Geometry check sheet. Reference: the model listing, model coordinates, mm. A direction names the side the tool comes from. Round coordinates to 2 decimals unless told otherwise and drop trailing zeros. Loops run counter-clockwise (first coordinate to the right, second up) from the corner with the lowest first, then second, coordinate; pieces in that order, holes last. Notation, with made-up numbers: (47, -8) - (83, -8) arc R23 cw to (83, 18) - close; hole circle Ø7 at (29.5, -4). An arc over 180 degrees is marked (long way). Answer in a Markdown table with one row per item. Add a question column.
```python
from build123d import *

# Parameters (mm, degrees)
F0_R     = 10
F1_DEPTH = 2
F2_R     = 4
F3_DEPTH = 0.5
F4_R     = 3.175
F5_DEPTH = 2
F6_R     = 9
F6_R_2   = 8
F6_R_3   = 7
F6_R_4   = 6
F6_R_5   = 5
F6_R_6   = 4
F7_DEPTH = 0.5
F8_SIZE2 = 0.49999
F8_SIZE  = 5.99999
F9_SIZE  = 0.5


# Not quite as in the source:
# - a fillet or chamfer is up to 0.001 mm smaller than in the source, because OpenCascade refuses the exact size


with BuildPart() as f1:
    # F0 (on Top) → F1 (new body)
    with BuildSketch(Plane.XY):
        Circle(F0_R)
    extrude(amount=F1_DEPTH)

    # F2 (on face) → F3 (join)
    with BuildSketch(Plane.XY.offset(2)):
        Circle(F2_R)
    extrude(amount=F3_DEPTH)

    # F4 (on face) → F5 (join)
    with BuildSketch(Plane.XY.offset(2.5)):
        Circle(F4_R)
    extrude(amount=F5_DEPTH)

    # F6 (on face) → F7 (cut)
    with BuildSketch(Plane(origin=(0, 0, 0), x_dir=(1, 0, 0), z_dir=(0, 0, -1))):
        Circle(F6_R)
        Circle(F6_R_2, mode=Mode.SUBTRACT)
        Circle(F6_R_3)
        Circle(F6_R_4, mode=Mode.SUBTRACT)
        Circle(F6_R_5)
        Circle(F6_R_6, mode=Mode.SUBTRACT)
    extrude(amount=-F7_DEPTH, mode=Mode.SUBTRACT)

    # F8 (size 6 and 0.5 in the source; OpenCascade refuses exactly that, so slightly less here)
    f8_edges = [f1.edges().sort_by_distance(p)[0] for p in [
        (-10, 0, 2),
    ]]
    f8_side = f1.faces().sort_by_distance((-9.717157, 0, 2))[0]
    chamfer(f8_edges, length=F8_SIZE, length2=F8_SIZE2, reference=f8_side)

    # F9
    f9_edges = [f1.edges().sort_by_distance(p)[0] for p in [
        (-3.175, 0, 4.5),
    ]]
    chamfer(f9_edges, length=F9_SIZE)


solid = f1.part
```
Q1. Cross-section at A-A, the plane z = 2.8. Enter the section's corners in (x, y) (3 decimals), plus the area to 3 significant figures.
Q2. Set-up check for faces 1 (the cylindrical face through (-0.69, -3.1, 3.24)), 2 (the flat face through (4, -6, 0)), 3 (the cylindrical face through (-1.08, 4.88, 0.25)): record each of +Z, -Z, +X, -X, +Y, -Y from which the full face is reachable in a straight line by a thin tool's end or side.
Q3. Depth check by flat-ended pin: P1, Ø9, axis at x = -2, y = -1, coming from the -Z side; P2, Ø2, axis at x = -1.5, z = 1, coming from the -Y side. Enter the tip coordinate at first touch or a pass-through.
Q4. Scan lines: line 1 (Z direction, x = 4, y = 0.75); line 2 (Z direction, x = -3.5, y = 0.25); line 3 (Y direction, x = 2.25, z = 2.7). Record each from-to range of solid material in increasing order. Write a range as from..to.
Q5. Release check for a two-part mould opening along X. For faces 4 (the conical face through (4.17, 1.31, 1.97)), 5 (the flat face through (-3, 2, 2.5)), 6 (the cylindrical face through (6.466, 2.681, 0.246)) record: +X half, -X half, draft (parallel to the pull), parting line (faces both ways), or undercut.
Check sheet entries:
| question | item | result |
|---|---|---|
| 1 | outline | circle Ø6.35 at (0, 0) |
| 1 | area | 31.7 mm² |
| 2 | face 1 | +Z |
| 2 | face 2 | -Z, +X, -X, +Y, -Y |
| 2 | face 3 | -Z |
| 3 | P1 | z = 0 |
| 3 | P2 | y = -9.99 |
| 4 | line 1 | 0.5..1.99 |
| 4 | line 2 | 0..2.5 |
| 4 | line 3 | -2.24..2.24 |
| 5 | face 4 | parting line |
| 5 | face 5 | draft |
| 5 | face 6 | undercut |
